For this review, take the finished solid that the model builds, in its own axes (mm). A direction names the side the tool comes from. Coordinates: 2 decimals unless noted, no trailing zeros. Loops run counter-clockwise (first coordinate to the right, second up) from the corner with the lowest first, then second, coordinate; pieces in that order, holes last. Notation, with made-up numbers: M -1.75,62 L 38.25,62 A25 cw 38.25,75 Z; hole C 70.5,66 d8. An arc over 180 degrees is marked long. Write each question's results on one line, items separated by ' | '. Start each with the question number.
Autodesk Inventor part; units mm, degrees
ref_plane "YZ Plane" through (0, 0, 0) normal (1, 0, 0) x (0, 1, 0)
ref_plane "XZ Plane" through (0, 0, 0) normal (0, 1, 0) x (-1, 0, 0)
ref_plane "XY Plane" through (0, 0, 0) normal (0, 0, 1) x (1, 0, 0)
sketch "スケッチ1" plane through (0, 0, 0) normal (0, 0, 1) x (1, 0, 0)
  line L0 (-28.5941, 8.0239) -> (-27.6141, 8.0239)
  line L1 (-27.6141, 8.0239) -> (-27.6141, 6.8739)
  line L2 (-27.6141, 6.8739) -> (-28.5941, 6.8739)
  line L3 (-28.5941, 6.8739) -> (-28.5941, 8.0239)
  line L4 (-23.6141, 8.0239) -> (-22.6341, 8.0239)
  line L5 (-22.6341, 8.0239) -> (-22.6341, 6.8739)
  line L6 (-22.6341, 6.8739) -> (-23.6141, 6.8739)
  line L7 (-23.6141, 6.8739) -> (-23.6141, 8.0239)
  line L8 (-18.6341, 8.0239) -> (-17.6541, 8.0239)
  line L9 (-17.6541, 8.0239) -> (-17.6541, 6.8739)
  line L10 (-17.6541, 6.8739) -> (-18.6341, 6.8739)
  line L11 (-18.6341, 6.8739) -> (-18.6341, 8.0239)
  line L12 (-28.5941, 3.2739) -> (-27.6141, 3.2739)
  line L13 (-27.6141, 3.2739) -> (-27.6141, 2.1239)
  line L14 (-27.6141, 2.1239) -> (-28.5941, 2.1239)
  line L15 (-28.5941, 2.1239) -> (-28.5941, 3.2739)
  line L16 (-23.6141, 3.2739) -> (-22.6341, 3.2739)
  line L17 (-22.6341, 3.2739) -> (-22.6341, 2.1239)
  line L18 (-22.6341, 2.1239) -> (-23.6141, 2.1239)
  line L19 (-23.6141, 2.1239) -> (-23.6141, 3.2739)
  line L20 (-18.6341, 3.2739) -> (-17.6541, 3.2739)
  line L21 (-17.6541, 3.2739) -> (-17.6541, 2.1239)
  line L22 (-17.6541, 2.1239) -> (-18.6341, 2.1239)
  line L23 (-18.6341, 2.1239) -> (-18.6341, 3.2739)
  dimension "d2" = 0.98
  dimension "d3" = 1.15
  dimension "d4" = 0.98
  dimension "d5" = 1.15
  dimension "d6" = 0.98
  dimension "d7" = 1.15
  dimension "d8" = 0.98
  dimension "d9" = 1.15
  dimension "d10" = 0.98
  dimension "d11" = 1.15
  dimension "d12" = 0.98
  dimension "d13" = 1.15
  dimension "d14" = 4
  dimension "d15" = 0
  dimension "d16" = 0
  dimension "d17" = 4
  dimension "d18" = 0
  dimension "d19" = 0
  dimension "d20" = 3.6
  dimension "d21" = 4
  dimension "d22" = 0
  dimension "d23" = 0
extrude "押し出し1" add sketch "スケッチ1" along normal blind 5
sketch "スケッチ2" plane through (0, 0, 5) normal (0, 0, 1) x (1, 0, 0)
  line L0 (-29.6241, 11.5739) -> (-16.6241, 11.5739)
  line L1 (-16.6241, 11.5739) -> (-16.6241, -1.4261)
  line L2 (-16.6241, -1.4261) -> (-29.6241, -1.4261)
  line L3 (-29.6241, -1.4261) -> (-29.6241, 11.5739)
  line L4 (-17.6541, 8.0239) -> (-18.6341, 8.0239)
  line L5 (-17.6541, 2.1239) -> (-17.6541, 3.2739)
  line L6 (-28.5941, 3.2739) -> (-28.5941, 2.1239)
  point P0 (0, 0)
  dimension "d26" = 13
  dimension "d27" = 13
  dimension "d28" = 3.55
  dimension "d29" = 10.94
  dimension "d30" = 1.03
extrude "押し出し2" add sketch "スケッチ2" along normal blind 10
equation "\"BendRadius\" = Thickness"
equation "\"BendReliefWidth\" = Thickness"
equation "\"BendReliefDepth\" = 0.5 * Thickness"
equation "\"CornerReliefSize\" = 4 * Thickness"
equation "\"MinimumRemnant\" = 2 * Thickness"
equation "\"TransitionRadius\" = BendRadius"
equation "\"JacobiRadiusSize\" = BendRadius"
equation "\"GapSize\" = Thickness"
properties part number "pin"
Q1. Take a section at A-A, the plane z = 2.5. Give the boundary of the cut face in (x, y), then the cut area to 3 significant figures.
Q2. Take a section at D-D, the plane x = -21. Give the boundary of the cut face in (y, z), then the cut area to 3 significant figures.
Q3. Take a section at C-C, the plane y = 2.5. Give the boundary of the cut face in (x, z), then the cut area to 3 significant figures.
Q4. The part is to be moulded in two halves that separate along Y. For faces 1 (the face through (-23, 11.574, 10)), 2 (the face through (-27.614, 7.5, 2.5)), 3 (the face through (-28, 2.124, 2)), 4 (the face through (-23, 6.874, 2)), say which applies: pulls with the +Y half, pulls with the -Y half, needs draft (parallel to the pull), parting line crosses it, or undercut.
Q5. Insertion check: P1, Ø1.1, axis at x = -23.5, z = 3, coming from the -Y side; P2, Ø1.5, axis at x = -21, z = 4, coming from the +Y side; P3, Ø1.1, axis at x = -18, z = 2, coming from the +Y side; P4, Ø1.3, axis at y = 3, z = 2.5, coming from the +X side. Each pin has a flat end and moves straight along its axis. Give the tip position at first contact, or say it passes through.
Q6. To check wall thickness, follow line 1 along Y through (x, z) = (-23, 4); line 2 along Z through (x, y) = (-27, 8.75). State the ranges of each line that lie inside material, in increasing order.
Q7. Take a section at B-B, the plane x = -28.25. Give the boundary of the cut face in (y, z), then the cut area to 4 significant figures.
Q8. For faces 5 (the face through (-23.614, 3, 2)), 6 (the face through (-17.654, 3, 2)), 7 (the face through (-29.624, 5, 10)), 8 (the face through (-18, 2.124, 2)), 9 (the face through (-28.594, 3, 2)), list the 3-axis set-ups (+Z, -Z, +X, -X, +Y, -Y) from which the entire face can be reached by the end or side of a thin tool; tool diameter is ignored.
Results:
1) outline: M -28.59,2.12 L -27.61,2.12 L -27.61,3.27 L -28.59,3.27 Z; M -28.59,6.87 L -27.61,6.87 L -27.61,8.02 L -28.59,8.02 Z; M -23.61,2.12 L -22.63,2.12 L -22.63,3.27 L -23.61,3.27 Z; M -23.61,6.87 L -22.63,6.87 L -22.63,8.02 L -23.61,8.02 Z; M -18.63,2.12 L -17.65,2.12 L -17.65,3.27 L -18.63,3.27 Z; M -18.63,6.87 L -17.65,6.87 L -17.65,8.02 L -18.63,8.02 Z | area: 6.76 mm^2
2) outline: M -1.43,5 L 11.57,5 L 11.57,15 L -1.43,15 Z | area: 130 mm^2
3) outline: M -29.62,5 L -28.59,5 L -28.59,0 L -27.61,0 L -27.61,5 L -23.61,5 L -23.61,0 L -22.63,0 L -22.63,5 L -18.63,5 L -18.63,0 L -17.65,0 L -17.65,5 L -16.62,5 L -16.62,15 L -29.62,15 Z | area: 145 mm^2
4) face 1: pulls with the +Y half | face 2: needs draft | face 3: pulls with the -Y half | face 4: undercut
5) P1: y = 2.12 | P2: through | P3: y = 8.02 | P4: x = -17.65
6) line 1: 2.12 to 3.27, 6.87 to 8.02 | line 2: 5 to 15
7) outline: M -1.43,5 L 2.12,5 L 2.12,0 L 3.27,0 L 3.27,5 L 6.87,5 L 6.87,0 L 8.02,0 L 8.02,5 L 11.57,5 L 11.57,15 L -1.43,15 Z | area: 141.5 mm^2
8) face 5: -Z, +Y, -Y | face 6: -Z, +X, +Y, -Y | face 7: +Z, -Z, -X, +Y, -Y | face 8: -Z, +X, -X, -Y | face 9: -Z, -X, +Y, -Y
